Verification items for the finished model (mm, model axes). Coordinates: 2 decimals unless noted, no trailing zeros.
Q1. Cross-section at A-A, the plane z = 1.6. Count the separate pieces of the cut face and the enclosed holes in it, and give its area (3 significant figures).
Q2. Depth check by flat-ended pin: P1, Ø8, axis at x = 50, y = 86.6, coming from the +Z side; P2, Ø0.9, axis at x = -42.5, z = 2, coming from the +Y side; P3, Ø1.5, axis at x = -96.5, z = 1, coming from the +Y side. Enter the tip coordinate at first touch or a pass-through.
Q3. Thickness scan on line 1 (X direction, y = 25, z = 1.9); line 2 (Y direction, x = -61, z = 2.7); line 3 (Y direction, x = 33, z = 2.15). Record the ranges inside material, lowest first.
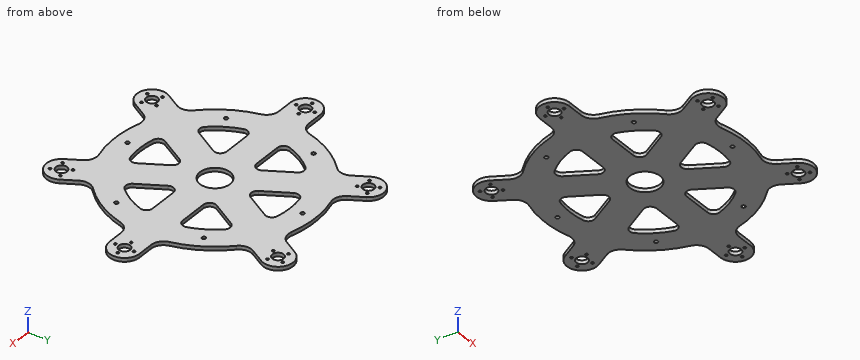
from build123d import *

# Parameters (mm, degrees)
SKETCH1_R           = 4.5
SKETCH1_R_2         = 1
SKETCH1_R_3         = 12
SKETCH1_R_4         = 1.5
BOSS_EXTRUDE1_DEPTH = 3


with BuildPart() as part:
    # Sketch1 → Boss-Extrude1 (new body)
    with BuildSketch(Plane.XY):
        with BuildLine():
            Line((-54.027153304, 69.577774511), (-60.392304845, 80.602540378))
            ThreePointArc((-60.392304845, 80.602540378), (-56, 96.994845224), (-39.607695155, 92.602540378))
            Line((-39.607695155, 92.602540378), (-33.242543613, 81.577774511))
            ThreePointArc((-33.242543613, 81.577774511), (-28.3404086, 77.310814848), (-21.850924067, 76.958021787))
            ThreePointArc((-21.850924067, 76.958021787), (0, 80), (21.850924067, 76.958021787))
            ThreePointArc((21.850924067, 76.958021787), (28.3404086, 77.310814848), (33.242543613, 81.577774511))
            Line((33.242543613, 81.577774511), (39.607695155, 92.602540378))
            ThreePointArc((39.607695155, 92.602540378), (56, 96.994845224), (60.392304845, 80.602540378))
            Line((60.392304845, 80.602540378), (54.027153304, 69.577774511))
            ThreePointArc((54.027153304, 69.577774511), (52.782925345, 63.198921225), (55.722139859, 57.402466232))
            ThreePointArc((55.722139859, 57.402466232), (69.282032303, 40), (77.573063926, 19.555555556))
            ThreePointArc((77.573063926, 19.555555556), (81.123333946, 14.111893623), (87.269696917, 12))
            Line((87.269696917, 12), (100, 12))
            ThreePointArc((100, 12), (112, 0), (100, -12))
            Line((100, -12), (87.269696917, -12))
            ThreePointArc((87.269696917, -12), (81.123333946, -14.111893623), (77.573063926, -19.555555556))
            ThreePointArc((77.573063926, -19.555555556), (69.282032303, -40), (55.722139859, -57.402466232))
            ThreePointArc((55.722139859, -57.402466232), (52.782925345, -63.198921225), (54.027153304, -69.577774511))
            Line((54.027153304, -69.577774511), (60.392304845, -80.602540378))
            ThreePointArc((60.392304845, -80.602540378), (56, -96.994845224), (39.607695155, -92.602540378))
            Line((39.607695155, -92.602540378), (33.242543613, -81.577774511))
            ThreePointArc((33.242543613, -81.577774511), (28.3404086, -77.310814848), (21.850924067, -76.958021787))
            ThreePointArc((21.850924067, -76.958021787), (0, -80), (-21.850924067, -76.958021787))
            ThreePointArc((-21.850924067, -76.958021787), (-28.3404086, -77.310814848), (-33.242543613, -81.577774511))
            Line((-33.242543613, -81.577774511), (-39.607695155, -92.602540378))
            ThreePointArc((-39.607695155, -92.602540378), (-56, -96.994845224), (-60.392304845, -80.602540378))
            Line((-60.392304845, -80.602540378), (-54.027153304, -69.577774511))
            ThreePointArc((-54.027153304, -69.577774511), (-52.782925345, -63.198921225), (-55.722139859, -57.402466232))
            ThreePointArc((-55.722139859, -57.402466232), (-69.282032303, -40), (-77.573063926, -19.555555556))
            ThreePointArc((-77.573063926, -19.555555556), (-81.123333946, -14.111893623), (-87.269696917, -12))
            Line((-87.269696917, -12), (-100, -12))
            ThreePointArc((-100, -12), (-112, 0), (-100, 12))
            Line((-100, 12), (-87.269696917, 12))
            ThreePointArc((-87.269696917, 12), (-81.123333946, 14.111893623), (-77.573063926, 19.555555556))
            ThreePointArc((-77.573063926, 19.555555556), (-69.282032303, 40), (-55.722139859, 57.402466232))
            ThreePointArc((-55.722139859, 57.402466232), (-52.782925345, 63.198921225), (-54.027153304, 69.577774511))
        make_face()
        with Locations((100, 0)):
            Circle(SKETCH1_R, mode=Mode.SUBTRACT)
        with Locations((107.425, 0)):
            Circle(SKETCH1_R_2, mode=Mode.SUBTRACT)
        with Locations((100, 7.425)):
            Circle(SKETCH1_R_2, mode=Mode.SUBTRACT)
        with Locations((92.575, 0)):
            Circle(SKETCH1_R_2, mode=Mode.SUBTRACT)
        with Locations((100, -7.425)):
            Circle(SKETCH1_R_2, mode=Mode.SUBTRACT)
        with Locations((50, -86.602540378)):
            Circle(SKETCH1_R, mode=Mode.SUBTRACT)
        with Locations((56.430238623, -82.890040378)):
            Circle(SKETCH1_R_2, mode=Mode.SUBTRACT)
        with Locations((53.7125, -93.032779002)):
            Circle(SKETCH1_R_2, mode=Mode.SUBTRACT)
        with Locations((43.569761377, -90.315040378)):
            Circle(SKETCH1_R_2, mode=Mode.SUBTRACT)
        with Locations((46.2875, -80.172301755)):
            Circle(SKETCH1_R_2, mode=Mode.SUBTRACT)
        with Locations((-50, -86.602540378)):
            Circle(SKETCH1_R, mode=Mode.SUBTRACT)
        with Locations((-43.569761377, -90.315040378)):
            Circle(SKETCH1_R_2, mode=Mode.SUBTRACT)
        with Locations((-53.7125, -93.032779002)):
            Circle(SKETCH1_R_2, mode=Mode.SUBTRACT)
        with Locations((-56.430238623, -82.890040378)):
            Circle(SKETCH1_R_2, mode=Mode.SUBTRACT)
        with Locations((-46.2875, -80.172301755)):
            Circle(SKETCH1_R_2, mode=Mode.SUBTRACT)
        with Locations((-100, 0)):
            Circle(SKETCH1_R, mode=Mode.SUBTRACT)
        with Locations((-100, -7.425)):
            Circle(SKETCH1_R_2, mode=Mode.SUBTRACT)
        with Locations((-107.425, 0)):
            Circle(SKETCH1_R_2, mode=Mode.SUBTRACT)
        with Locations((-100, 7.425)):
            Circle(SKETCH1_R_2, mode=Mode.SUBTRACT)
        with Locations((-92.575, 0)):
            Circle(SKETCH1_R_2, mode=Mode.SUBTRACT)
        with Locations((-50, 86.602540378)):
            Circle(SKETCH1_R, mode=Mode.SUBTRACT)
        with Locations((-56.430238623, 82.890040378)):
            Circle(SKETCH1_R_2, mode=Mode.SUBTRACT)
        with Locations((-53.7125, 93.032779002)):
            Circle(SKETCH1_R_2, mode=Mode.SUBTRACT)
        with Locations((-43.569761377, 90.315040378)):
            Circle(SKETCH1_R_2, mode=Mode.SUBTRACT)
        with Locations((-46.2875, 80.172301755)):
            Circle(SKETCH1_R_2, mode=Mode.SUBTRACT)
        with Locations((50, 86.602540378)):
            Circle(SKETCH1_R, mode=Mode.SUBTRACT)
        with Locations((43.569761377, 90.315040378)):
            Circle(SKETCH1_R_2, mode=Mode.SUBTRACT)
        with Locations((53.7125, 93.032779002)):
            Circle(SKETCH1_R_2, mode=Mode.SUBTRACT)
        with Locations((56.430238623, 82.890040378)):
            Circle(SKETCH1_R_2, mode=Mode.SUBTRACT)
        with Locations((46.2875, 80.172301755)):
            Circle(SKETCH1_R_2, mode=Mode.SUBTRACT)
        Circle(SKETCH1_R_3, mode=Mode.SUBTRACT)
        with Locations((0, 70)):
            Circle(SKETCH1_R_4, mode=Mode.SUBTRACT)
        with Locations((60.621778265, 35)):
            Circle(SKETCH1_R_4, mode=Mode.SUBTRACT)
        with Locations((60.621778265, -35)):
            Circle(SKETCH1_R_4, mode=Mode.SUBTRACT)
        with Locations((0, -70)):
            Circle(SKETCH1_R_4, mode=Mode.SUBTRACT)
        with Locations((-60.621778265, -35)):
            Circle(SKETCH1_R_4, mode=Mode.SUBTRACT)
        with Locations((-60.621778265, 35)):
            Circle(SKETCH1_R_4, mode=Mode.SUBTRACT)
        with BuildLine():
            Line((-36.545698507, 39.299006612), (-25.11473671, 19.5))
            ThreePointArc((-25.11473671, 19.5), (-25.11473671, 14.5), (-29.444863729, 12))
            Line((-29.444863729, 12), (-52.306787322, 12))
            ThreePointArc((-52.306787322, 12), (-56.351986497, 14.061230932), (-57.061949806, 18.545454545))
            ThreePointArc((-57.061949806, 18.545454545), (-51.961524227, 30), (-44.591809664, 40.144370849))
            ThreePointArc((-44.591809664, 40.144370849), (-40.353376444, 41.771636394), (-36.545698507, 39.299006612))
        make_face(mode=Mode.SUBTRACT)
        with BuildLine():
            Line((15.761088816, 51.299006612), (4.330127019, 31.5))
            ThreePointArc((4.330127019, 31.5), (0, 29), (-4.330127019, 31.5))
            Line((-4.330127019, 31.5), (-15.761088816, 51.299006612))
            ThreePointArc((-15.761088816, 51.299006612), (-15.998610053, 55.832867326), (-12.470140142, 58.689825394))
            ThreePointArc((-12.470140142, 58.689825394), (0, 60), (12.470140142, 58.689825394))
            ThreePointArc((12.470140142, 58.689825394), (15.998610053, 55.832867326), (15.761088816, 51.299006612))
        make_face(mode=Mode.SUBTRACT)
        with BuildLine():
            Line((36.545698507, 39.299006612), (25.11473671, 19.5))
            ThreePointArc((25.11473671, 19.5), (25.11473671, 14.5), (29.444863729, 12))
            Line((29.444863729, 12), (52.306787322, 12))
            ThreePointArc((52.306787322, 12), (56.351986497, 14.061230932), (57.061949806, 18.545454545))
            ThreePointArc((57.061949806, 18.545454545), (51.961524227, 30), (44.591809664, 40.144370849))
            ThreePointArc((44.591809664, 40.144370849), (40.353376444, 41.771636394), (36.545698507, 39.299006612))
        make_face(mode=Mode.SUBTRACT)
        with BuildLine():
            Line((52.306787322, -12), (29.444863729, -12))
            ThreePointArc((29.444863729, -12), (25.11473671, -14.5), (25.11473671, -19.5))
            Line((25.11473671, -19.5), (36.545698507, -39.299006612))
            ThreePointArc((36.545698507, -39.299006612), (40.353376444, -41.771636394), (44.591809664, -40.144370849))
            ThreePointArc((44.591809664, -40.144370849), (51.961524227, -30), (57.061949806, -18.545454545))
            ThreePointArc((57.061949806, -18.545454545), (56.351986497, -14.061230932), (52.306787322, -12))
        make_face(mode=Mode.SUBTRACT)
        with BuildLine():
            Line((15.761088816, -51.299006612), (4.330127019, -31.5))
            ThreePointArc((4.330127019, -31.5), (0, -29), (-4.330127019, -31.5))
            Line((-4.330127019, -31.5), (-15.761088816, -51.299006612))
            ThreePointArc((-15.761088816, -51.299006612), (-15.998610053, -55.832867326), (-12.470140142, -58.689825395))
            ThreePointArc((-12.470140142, -58.689825395), (0, -60), (12.470140142, -58.689825394))
            ThreePointArc((12.470140142, -58.689825394), (15.998610053, -55.832867326), (15.761088816, -51.299006612))
        make_face(mode=Mode.SUBTRACT)
        with BuildLine():
            Line((-36.545698507, -39.299006612), (-25.11473671, -19.5))
            ThreePointArc((-25.11473671, -19.5), (-25.11473671, -14.5), (-29.444863729, -12))
            Line((-29.444863729, -12), (-52.306787322, -12))
            ThreePointArc((-52.306787322, -12), (-56.351986497, -14.061230932), (-57.061949806, -18.545454545))
            ThreePointArc((-57.061949806, -18.545454545), (-51.961524227, -30), (-44.591809664, -40.144370849))
            ThreePointArc((-44.591809664, -40.144370849), (-40.353376444, -41.771636394), (-36.545698507, -39.299006612))
        make_face(mode=Mode.SUBTRACT)
    extrude(amount=BOSS_EXTRUDE1_DEPTH)


solid = part.part
Check values:
1. separate pieces: 1
1. enclosed holes: 43
1. area: 19,600 mm2
2. P1: passes through
2. P2: stops at y = 96.31
2. P3: stops at y = 12
3. line 1: x = -75.99 to -54.54, -28.29 to 28.29, 54.54 to 75.99
3. line 2: y = -91.4 to -81.81, -51.76 to -36.45, -33.55 to 33.55, 36.45 to 51.76, 81.81 to 91.4
3. line 3: y = -81.18 to -33.16, -12 to 12, 33.16 to 81.18
